from build123d import *

# Parameters (mm, degrees)
F0_W     = 25
F0_H     = 25
F1_DEPTH = 25
F2_R     = 7.5
F3_DEPTH = 15
F4_R     = 7.5
F5_DEPTH = 15


with BuildPart() as f1:
    # F0 (on Front) → F1 (new body)
    with BuildSketch(Plane.XZ):
        with Locations((12.5, 12.5)):
            Rectangle(F0_W, F0_H)
    extrude(amount=F1_DEPTH)

    # F2 (on Top) → F3 (join)
    with BuildSketch(Plane.XY):
        with Locations((12.704089, -11.857167)):
            Circle(F2_R)
    extrude(amount=-F3_DEPTH)

    # F4 (on face) → F5 (join)
    with BuildSketch(Plane.XY.offset(25)):
        with Locations((11.222606, -12.241699)):
            Circle(F4_R)
    extrude(amount=F5_DEPTH)


solid = f1.part
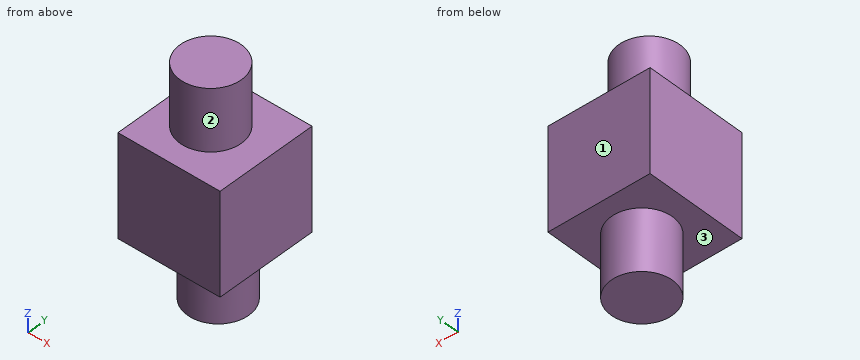
Geometry check sheet. Reference: the model listing, model coordinates, mm. Face numbers are marked on the shaded views. A direction names the side the tool comes from. Round coordinates to 2 decimals unless told otherwise and drop trailing zeros. Loops run counter-clockwise (first coordinate to the right, second up) from the corner with the lowest first, then second, coordinate; pieces in that order, holes last.
Item 1: Cross-section at C-C on y = -22.5. Record the boundary of the cut face in (x, z).
Item 2: Thickness scan on line 1 (Z direction, x = 8.75, y = -3); line 2 (Z direction, x = 7.75, y = -5.75); line 3 (X direction, y = -9, z = -4.5). Record the ranges inside material, lowest first.
Item 3: Cross-section at B-B on y = -17. Record the boundary of the cut face in (x, z), then the cut area to 3 significant figures.
Item 4: Cross-section at A-A on x = 6.25. Record the boundary of the cut face in (y, z), then the cut area to 3 significant figures.
Item 5: Access from +Z, -Z, +X, -X, +Y, -Y to the whole of each face (thin tool, end or side, straight path). Record for the marked faces 1, 2 and 3.
Item 6: Gauge pin test, flat ends, axial feed: pin 1 (1.5 mm diameter, centred on x = 12, y = -20.5, fed in from +Z); pin 2 (5 mm diameter, centred on x = 4.5, y = -3.5, fed in from -Z); pin 3 (1.5 mm diameter, centred on x = 13, z = 29.5, fed in from -Y). Record the tip position at first contact, or that the pin passes through.
Item 7: Cross-section at D-D on z = 31. Record the boundary of the cut face in (x, y).
Answer sheet:
1. outline: (0, 0) - (25, 0) - (25, 25) - (0, 25) - close
2. line 1: z = 0 to 25
2. line 2: z = 0 to 40
2. line 3: x = 5.77 to 19.64
3. outline: (0, 0) - (7.25, 0) - (7.25, -15) - (18.16, -15) - (18.16, 0) - (25, 0) - (25, 25) - (17.02, 25) - (17.02, 40) - (5.43, 40) - (5.43, 25) - (0, 25) - close
3. area: 963 mm2
4. outline: (-25, 0) - (-15.68, 0) - (-15.68, -15) - (-8.04, -15) - (-8.04, 0) - (0, 0) - (0, 25) - (-6.63, 25) - (-6.63, 40) - (-17.86, 40) - (-17.86, 25) - (-25, 25) - close
4. area: 908 mm2
5. face 1: +Z, -Z, +X, -X, +Y
5. face 2: +Z
5. face 3: -Z
6. pin 1: stops at z = 25
6. pin 2: stops at z = 0
6. pin 3: stops at y = -19.67
7. outline: circle Ø15 at (11.22, -12.24)
